from build123d import *

# Parameters (mm, degrees)
SKETCH1_W           = 6
SKETCH1_H           = 10
BOSS_EXTRUDE1_DEPTH = 13
SKETCH2_W           = 4
SKETCH2_H           = 6
CUT_EXTRUDE1_DEPTH  = 11
SKETCH3_W           = 10
SKETCH3_H           = 4
BOSS_EXTRUDE2_DEPTH = 2
LPATTERN1_COUNT     = 2
LPATTERN1_PITCH     = 8
SKETCH18_W          = 10
SKETCH18_H          = 8
BOSS_EXTRUDE3_DEPTH = 8
SKETCH20_W          = 10
SKETCH20_H          = 4
BOSS_EXTRUDE4_DEPTH = 2
SKETCH21_W          = 10
SKETCH21_H          = 8
BOSS_EXTRUDE5_DEPTH = 6
SKETCH22_W          = 40
SKETCH22_H          = 8
BOSS_EXTRUDE6_DEPTH = 2
SKETCH23_W          = 4
SKETCH23_H          = 6
CUT_EXTRUDE2_DEPTH  = 6


with BuildPart() as part:
    # Sketch1 → Boss-Extrude1 (new body)
    with BuildSketch(Plane(origin=(0, 0, 0), x_dir=(1, 0, 0), z_dir=(0, 1, 0))):
        with Locations((3, 5)):
            Rectangle(SKETCH1_W, SKETCH1_H)
    extrude(amount=BOSS_EXTRUDE1_DEPTH)

    # Sketch2 → Cut-Extrude1 (cut)
    with BuildSketch(Plane.XZ):
        with Locations((3, -5)):
            Rectangle(SKETCH2_W, SKETCH2_H)
    extrude(amount=-CUT_EXTRUDE1_DEPTH, mode=Mode.SUBTRACT)

    # Sketch3 → Boss-Extrude2 (add)
    with BuildSketch(Plane.ZY):
        with Locations((-5, 2)):
            Rectangle(SKETCH3_W, SKETCH3_H)
    extrude(amount=BOSS_EXTRUDE2_DEPTH)


with BuildPart() as lpattern1_1:
    # LPattern1: pattern copy
    add(part.part.moved(Location(Vector(-1, 0, 0) * (1 * LPATTERN1_PITCH))))

    # Sketch18 → Boss-Extrude3 (add)
    with BuildSketch(Plane.ZY.offset(10)):
        with Locations((-5, 4)):
            Rectangle(SKETCH18_W, SKETCH18_H)
    extrude(amount=BOSS_EXTRUDE3_DEPTH)


with BuildPart() as part_1:
    add(part.part)

    # Sketch20 → Boss-Extrude4 (add)
    with BuildSketch(Plane(origin=(6, 0, 0), x_dir=(0, 0, -1), z_dir=(1, 0, 0))):
        with Locations((5, 2)):
            Rectangle(SKETCH20_W, SKETCH20_H)
    extrude(amount=BOSS_EXTRUDE4_DEPTH)

    # Sketch21 → Boss-Extrude5 (add)
    with BuildSketch(Plane(origin=(8, 0, 0), x_dir=(0, 0, -1), z_dir=(1, 0, 0))):
        with Locations((5, 4)):
            Rectangle(SKETCH21_W, SKETCH21_H)
    extrude(amount=BOSS_EXTRUDE5_DEPTH)

    # Sketch22 → Boss-Extrude6 (add)
    with BuildSketch(Plane(origin=(14, 0, 0), x_dir=(0, 0, -1), z_dir=(1, 0, 0))):
        with Locations((5, 4)):
            Rectangle(SKETCH22_W, SKETCH22_H)
    extrude(amount=BOSS_EXTRUDE6_DEPTH)


with BuildPart() as cut_extrude2_tool:
    # Sketch23 → Cut-Extrude2 (new body)
    with BuildSketch(Plane.XZ):
        with Locations((11, -5)):
            Rectangle(SKETCH23_W, SKETCH23_H)
        with Locations((-13, -5)):
            Rectangle(SKETCH23_W, SKETCH23_H)
    extrude(amount=-CUT_EXTRUDE2_DEPTH)


with BuildPart() as part_2:
    add(part_1.part)

    # Cut-Extrude2: cut by cut_extrude2_tool
    add(cut_extrude2_tool.part, mode=Mode.SUBTRACT)


with BuildPart() as lpattern1_1_1:
    add(lpattern1_1.part)

    # Cut-Extrude2: cut by cut_extrude2_tool
    add(cut_extrude2_tool.part, mode=Mode.SUBTRACT)

    # Combine1: union part
    add(part_2.part)


solid = lpattern1_1_1.part
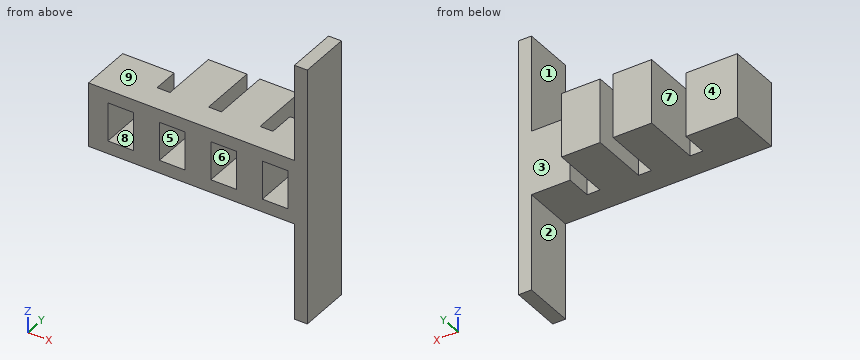
Input: part model. Units: mm. Frame: model coordinates. Face numbers are marked on the shaded views. A direction names the side the tool comes from. Round coordinates to 2 decimals unless told otherwise and drop trailing zeros. Loops run counter-clockwise (first coordinate to the right, second up) from the corner with the lowest first, then second, coordinate; pieces in that order, holes last. Notation, with made-up numbers: M -26,73 L -12,73 A27 cw -12,110 Z; hole C 89.25,-34 d4. An arc over 180 degrees is marked long. Answer as CSV lines item,"result". Start each with the question number.
(1) Section D-D, the plane x = 12. Output: boundary loops of the cut face in (y, z), plus the area to 3 significant figures.
(2) Draft query along Z for the marked faces 6, 7, 8 and 9. Return one class per face: released by +Z, released by -Z, zero draft, split by the parting line, or undercut.
(3) Line query: line 1 (X direction, y = 10, z = -4.5); line 2 (X direction, y = 1, z = -2.5); line 3 (Z direction, x = 1.5, y = 3.75). Output: solid intervals per line, ascending. Write a range as [from, to].
(4) Reachability of the marked faces 1, 2, 3, 4 and 5 from +Z, -Z, +X, -X, +Y, -Y: full face, straight path, thin tool, end or side. Return the list, or none.
(5) Section C-C, the plane y = 1.75. Output: boundary loops of the cut face in (x, z).
(6) Section B-B, the plane y = 12. Output: boundary loops of the cut face in (x, z).
(7) Section A-A, the plane y = 8.5. Output: boundary loops of the cut face in (x, z), plus the area to 3 significant figures.
(8) First-contact query: pin 1 (6 mm diameter, centred on x = 9.5, z = -15.5, fed in from -Y); pin 2 (3 mm diameter, centred on x = -5, y = 4.5, fed in from -Z); pin 3 (6 mm diameter, centred on x = 4.5, y = 1.5, fed in from +Z); pin 4 (4 mm diameter, centred on y = 2.5, z = 4.5, fed in from -X). Flat tips, straight axial feed; report the tip coordinate or a pass-through.
Values found:
1,outline,"M 0,-10 L 8,-10 L 8,0 L 0,0 L 0,-2 L 6,-2 L 6,-8 L 0,-8 Z"
1,area,"44.0 mm²"
2,face 6,"undercut"
2,face 7,"zero draft"
2,face 8,"undercut"
2,face 9,"released by +Z"
3,line 1,"x = [-8, -7], [-3, -2], [0, 1], [5, 6]"
3,line 2,"x = [-18, -15], [-11, -7], [-3, 1], [5, 9], [13, 16]"
3,line 3,"z = [-10, -8], [-2, 0]"
4,face 1,"+Z, -X, +Y, -Y"
4,face 2,"-Z, -X, +Y, -Y"
4,face 3,"+Z, -Z, +X, +Y"
4,face 4,"+Z, -Z, -X, +Y"
4,face 5,"-Y"
5,outline,"M -18,-10 L 14,-10 L 14,-25 L 16,-25 L 16,15 L 14,15 L 14,0 L -18,0 Z; hole M -15,-8 L -11,-8 L -11,-2 L -15,-2 Z; hole M -7,-8 L -3,-8 L -3,-2 L -7,-2 Z; hole M 1,-8 L 5,-8 L 5,-2 L 1,-2 Z; hole M 9,-8 L 13,-8 L 13,-2 L 9,-2 Z"
6,outline,"M -8,-10 L -2,-10 L -2,0 L -8,0 Z; M 0,-10 L 6,-10 L 6,0 L 0,0 Z"
7,outline,"M -8,-10 L -2,-10 L -2,0 L -8,0 Z; M 0,-10 L 6,-10 L 6,0 L 0,0 Z; hole M -7,-8 L -3,-8 L -3,-2 L -7,-2 Z; hole M 1,-8 L 5,-8 L 5,-2 L 1,-2 Z"
7,area,"72.0 mm²"
8,pin 1,"passes through"
8,pin 2,"stops at z = -10"
8,pin 3,"stops at z = 0"
8,pin 4,"stops at x = 14"
